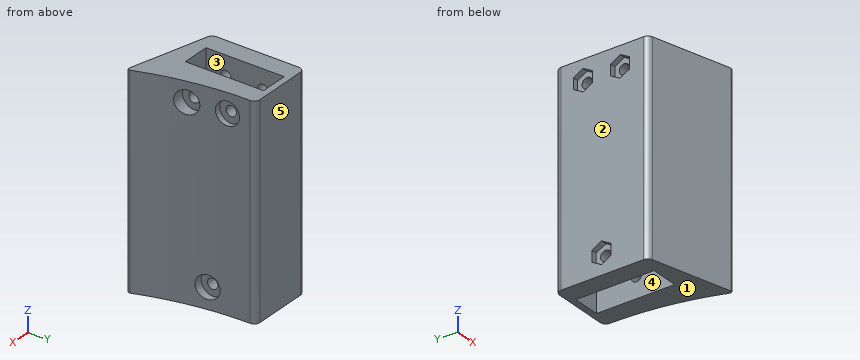
from build123d import *

# Parameters (mm, degrees)
ESQUISSE1_W             = 14.54
ESQUISSE1_H             = 40.8
BOSS_EXTRU_1_DEPTH      = 108
D_GAGEMENT_M1_62_D      = 5.4
CONG_1_R                = 3
CONG_2_R                = 1
ESQUISSE6_R             = 6
ENL_V_MAT_EXTRU_1_DEPTH = 15
ENL_V_MAT_EXTRU_2_DEPTH = 3


with BuildPart() as part:
    # Esquisse1 → Boss.-Extru.1 (new body)
    with BuildSketch(Plane.XY):
        with BuildLine():
            Line((-17.27, 44.084778495), (-17.27, -4.260431004))
            Line((-17.27, -4.260431004), (27.460015919, -16.245802647))
            ThreePointArc((27.460015919, -16.245802647), (19.521650941, 13.439236404), (17.27, 44.084778495))
            Line((17.27, 44.084778495), (-17.27, 44.084778495))
        make_face()
        with Locations((0, 20.4)):
            Rectangle(ESQUISSE1_W, ESQUISSE1_H, mode=Mode.SUBTRACT)
    extrude(amount=BOSS_EXTRU_1_DEPTH)

    # Dégagement M1.62 (through all)
    with Locations(Plane.ZY.offset(17.27)):
        with Locations((10.872493666, 20), (97.844217786, 29.700422986), (97.844217786, 10.299577014)):
            Hole(D_GAGEMENT_M1_62_D / 2)

    # Congé1
    cong_1_edges = [part.edges().sort_by_distance(p)[0] for p in [
        (17.27, 44.084778495, 54),
        (-17.27, -4.260431004, 54),
        (-17.27, 44.084778495, 54),
    ]]
    fillet(cong_1_edges, radius=CONG_1_R)

    # Congé2
    cong_2_edges = [part.edges().sort_by_distance(p)[0] for p in [
        (27.460015919, -16.245802647, 54),
    ]]
    fillet(cong_2_edges, radius=CONG_2_R)

    # Esquisse6 → Enlèv. mat.-Extru.1 (cut)
    with BuildSketch(Plane(origin=(30, 0, 0), x_dir=(0, 0, -1), z_dir=(1, 0, 0))):
        with Locations((-10.872493666, 20)):
            Circle(ESQUISSE6_R)
        with Locations((-97.844217786, 29.700422986)):
            Circle(ESQUISSE6_R)
        with Locations((-97.844217786, 10.299577014)):
            Circle(ESQUISSE6_R)
    extrude(amount=-ENL_V_MAT_EXTRU_1_DEPTH, mode=Mode.SUBTRACT)

    # Esquisse7 → Enlèv. mat.-Extru.2 (cut)
    with BuildSketch(Plane.ZY.offset(17.27)):
        Polygon((13.759245012, 15), (16.645996358, 20), (13.759245012, 25), (7.98574232, 25), (5.098990974, 20), (7.98574232, 15), align=None)
        Polygon((100.730969132, 24.700422986), (103.617720477, 29.700422986), (100.730969132, 34.700422986), (94.95746644, 34.700422986), (92.070715094, 29.700422986), (94.95746644, 24.700422986), align=None)
        Polygon((100.730969132, 5.299577014), (103.617720477, 10.299577014), (100.730969132, 15.299577014), (94.95746644, 15.299577014), (92.070715094, 10.299577014), (94.95746644, 5.299577014), align=None)
    extrude(amount=-ENL_V_MAT_EXTRU_2_DEPTH, mode=Mode.SUBTRACT)


solid = part.part
The listing builds one solid part. Answer for the finished solid, in the listing's coordinates (mm). Face numbers are marked on the shaded views. A direction names the side the tool comes from. Round coordinates to 2 decimals unless told otherwise and drop trailing zeros. Loops run counter-clockwise (first coordinate to the right, second up) from the corner with the lowest first, then second, coordinate; pieces in that order, holes last. Notation, with made-up numbers: M 67.5,-9 L 103.5,-9 A18 cw 103.5,-2 Z; hole C -31,79 d8. An arc over 180 degrees is marked long. Write each question's results on one line, items separated by ' | '. Start each with the question number.
1) Determine the mould class of the marked faces 1, 2 and 3 for opening direction X: pulls with the +X half, pulls with the -X half, needs draft (parallel to the pull), parting line crosses it, or undercut.
2) Find section C-C on y = 3. Write down the section's boundary in (x, z), plus the area to 3 significant figures.
3) Find section B-B on x = 10. Write down the section's boundary in (y, z).
4) Which of the six approach directions +Z, -Z, +X, -X, +Y, -Y give full straight-line access (tool end or side, diameter ignored) to the marked faces 4 and 5?
5) Each of these flat-tipped pins is pushed along its axis until it touches: pin 1 (1.5 mm diameter, centred on x = -15.5, z = 96.5, fed in from -Y); pin 2 (2 mm diameter, centred on x = -12, z = 44, fed in from -Y); pin 3 (13 mm diameter, centred on y = 31, z = 100.5, fed in from +X). Where does it stop, or does it pass through?
6) Straight lines are drawn through the part: probe 1 along X at (y, z) = (36, 29); probe 2 along Y at (x, z) = (14, 95.5); probe 3 along X at (y, z) = (33, 30.5). For each, find the intervals that lie inside material, in ascending order.
7) Find section D-D on x = -5. Write down the section's boundary in (y, z), plus the area to 3 significant figures.
8) Find section A-A on z = 54.5. Write down the section's boundary in (x, y), plus the area to 3 significant figures.
Final values:
1) face 1: needs draft | face 2: pulls with the -X half | face 3: undercut
2) outline: M -17.27,0 L -7.27,0 L -7.27,108 L -17.27,108 Z; M 7.27,0 L 21.64,0 L 21.64,108 L 7.27,108 Z | area: 2,630 mm²
3) outline: M -11.57,0 L 44.08,0 L 44.08,108 L -11.57,108 Z; hole C 10.3,97.84 d5.4; hole C 20,10.87 d5.4; hole C 29.7,97.84 d5.4
4) face 4: +Z, -Z | face 5: +Z, -Z, +X, -X, +Y
5) pin 1: y = -4.94 | pin 2: y = -5.94 | pin 3: x = 18.04
6) probe 1: -17.27 to -7.27, 7.27 to 17.3 | probe 2: -12.64 to 8.96, 11.64 to 28.36, 31.04 to 44.08 | probe 3: -17.27 to -7.27, 7.27 to 17.42
7) outline: M -7.55,0 L 0,0 L 0,108 L -7.55,108 Z; M 40.8,0 L 44.08,0 L 44.08,108 L 40.8,108 Z | area: 1,170 mm²
8) outline: M -17.27,-1.96 A3 ccw -15.05,-4.86 L 25.6,-15.75 A1 ccw 26.8,-14.45 A163.72 cw 17.24,41.08 A3 ccw 14.24,44.08 L -14.27,44.08 A3 ccw -17.27,41.08 Z; hole M -7.27,0 L 7.27,0 L 7.27,40.8 L -7.27,40.8 Z | area: 1,410 mm²
